Source: three-view drawing plus pictorial views. Frame: mm from the lowest corner of the part. A direction names the side the tool comes from. Round coordinates to 2 decimals unless told otherwise and drop trailing zeros. Loops run counter-clockwise (first coordinate to the right, second up) from the corner with the lowest first, then second, coordinate; pieces in that order, holes last. Notation, with made-up numbers: (73.5, 63) -> (117.5, 63) arc R35 cw to (117.5, 97) -> close; hole circle Ø6 at (-8.5, 65.5). An arc over 180 degrees is marked (long way). Answer in a Markdown table with one row per item. Add a question column.
Q1. Ray query, L1, parallel to Y at x = 17, z = 63; L2, parallel to Z at x = 29.5, y = 20.5; L3, parallel to Z at x = 30, y = 5.5. Return the intervals inside material, ascending. Write a range as from..to.
Q2. Reachability of the marked faces 1, 2 and 3 from +Z, -Z, +X, -X, +Y, -Y: full face, straight path, thin tool, end or side. Return the list, or none.
Q3. Section C-C, the plane z = 48.5. Output: boundary loops of the cut face in (x, y).
Q4. Section B-B, the plane y = 4.5. Output: boundary loops of the cut face in (x, z).
Q5. Pin query (flat end, axial travel): pin 1 (4.5 mm diameter, centred on x = 17.5, z = 5.5, fed in from +Y); pin 2 (10 mm diameter, centred on y = 10.5, z = 36.5, fed in from -X); pin 3 (2 mm diameter, centred on x = 13, z = 35, fed in from +Y). Return the tip coordinate at first contact, or that it passes through.
Q6. Section A-A, the plane x = 17.5. Output: boundary loops of the cut face in (y, z).
Q7. Section D-D, the plane x = 27.5. Output: boundary loops of the cut face in (y, z), and give its area (3 significant figures).
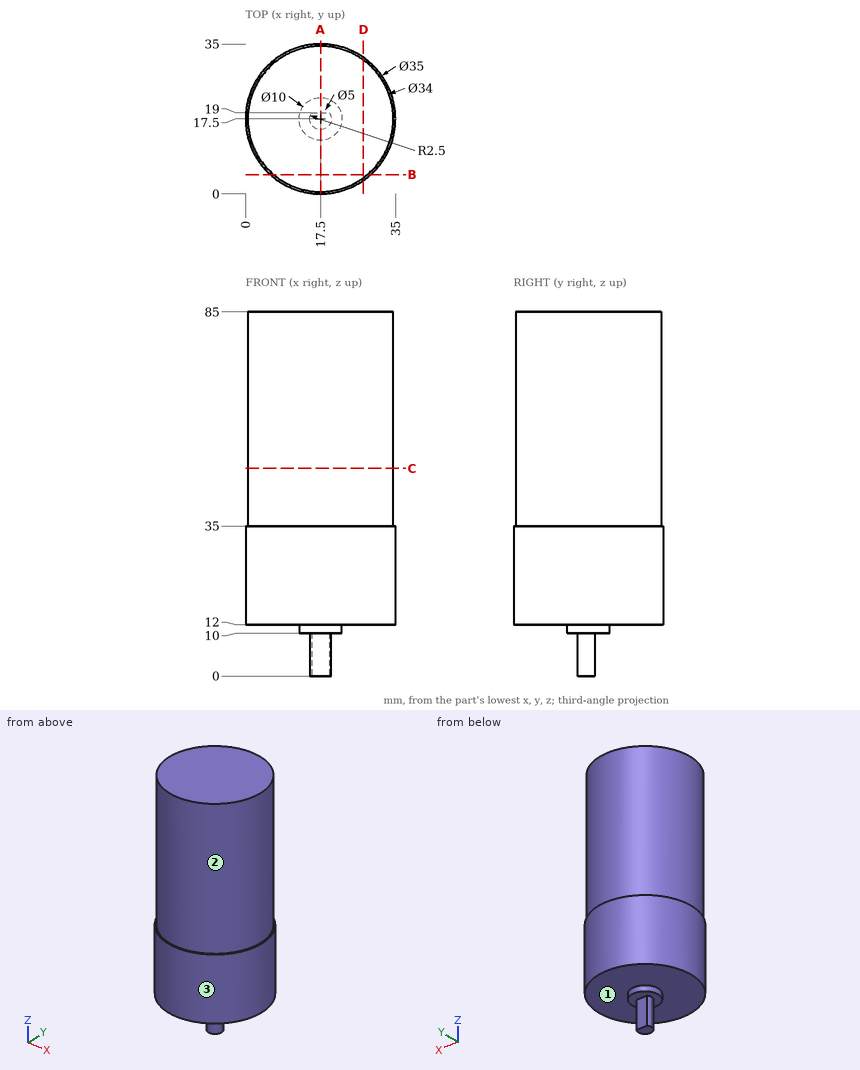
Answer block:
| question | item | result |
|---|---|---|
| 1 | L1 | 0.51..34.49 |
| 1 | L2 | 12..85 |
| 1 | L3 | 12..35 |
| 2 | face 1 | -Z |
| 2 | face 2 | +Z |
| 2 | face 3 | +Z, -Z |
| 3 | outline | circle Ø34 at (17.5, 17.5) |
| 4 | outline | (5.78, 12) -> (29.22, 12) -> (29.22, 35) -> (28.45, 35) -> (28.45, 85) -> (6.55, 85) -> (6.55, 35) -> (5.78, 35) -> close |
| 5 | pin 1 | y = 19 |
| 5 | pin 2 | x = 0.14 |
| 5 | pin 3 | y = 34.65 |
| 6 | outline | (0, 12) -> (12.5, 12) -> (12.5, 10) -> (15, 10) -> (15, 0) -> (19, 0) -> (19, 10) -> (22.5, 10) -> (22.5, 12) -> (35, 12) -> (35, 35) -> (34.5, 35) -> (34.5, 85) -> (0.5, 85) -> (0.5, 35) -> (0, 35) -> close |
| 7 | outline | (3.14, 12) -> (31.86, 12) -> (31.86, 35) -> (31.25, 35) -> (31.25, 85) -> (3.75, 85) -> (3.75, 35) -> (3.14, 35) -> close |
| 7 | area | 2,040 mm^2 |
